```python
from build123d import *

# Parameters (mm, degrees)
SKETCH1_R               = 1.7526
BOSS_EXTRUDE1_DEPTH     = 20.240625
CUT_EXTRUDE1_START      = 17.4625
CUT_EXTRUDE1_DEPTH      = 6.35
CUT_EXTRUDE2_START      = -17.4625
CUT_EXTRUDE2_DEPTH      = 6.35
CUT_EXTRUDE3_DEPTH      = 40.737078408
CUT_EXTRUDE3_DEPTH_BACK = 40.737078408
SKETCH4_R               = 15.875


with BuildPart() as part:
    # Sketch1 → Boss-Extrude1 (new, symmetric)
    with BuildSketch(Plane.XY):
        with BuildLine():
            Line((0, 31.75), (12.7, 31.75))
            ThreePointArc((12.7, 31.75), (3.690995675, 0), (12.7, -31.75))
            Line((12.7, -31.75), (0, -31.75))
            ThreePointArc((0, -31.75), (-9.009004325, 0), (0, 31.75))
        make_face()
        with Locations((3.690995675, 25.4)):
            Circle(SKETCH1_R, mode=Mode.SUBTRACT)
        with Locations((3.690995675, -25.4)):
            Circle(SKETCH1_R, mode=Mode.SUBTRACT)
    extrude(amount=BOSS_EXTRUDE1_DEPTH, both=True)

    # Sketch2 → Cut-Extrude1 (cut)
    with BuildSketch(Plane.XY.offset(CUT_EXTRUDE1_START)):
        Polygon((21.851555668, 28.575), (1.85790857, 28.575), (0.024821465, 25.4), (1.85790857, 22.225), (21.851555668, 22.225), align=None)
        Polygon((21.851555668, -28.575), (21.851555668, -22.225), (1.85790857, -22.225), (0.024821465, -25.4), (1.85790857, -28.575), align=None)
    extrude(amount=-CUT_EXTRUDE1_DEPTH, mode=Mode.SUBTRACT)

    # Sketch2<2> → Cut-Extrude2 (cut)
    with BuildSketch(Plane.XY.offset(CUT_EXTRUDE2_START)):
        Polygon((21.851555668, 28.575), (1.85790857, 28.575), (0.024821465, 25.4), (1.85790857, 22.225), (21.851555668, 22.225), align=None)
        Polygon((21.851555668, -28.575), (21.851555668, -22.225), (1.85790857, -22.225), (0.024821465, -25.4), (1.85790857, -28.575), align=None)
    extrude(amount=CUT_EXTRUDE2_DEPTH, mode=Mode.SUBTRACT)

    # Sketch4 → Cut-Extrude3 (cut, two sides: drawn at the far end of the back side and taken through both)
    with BuildSketch(Plane(origin=(0, 0, 0), x_dir=(0, 0, -1), z_dir=(1, 0, 0)).offset(-CUT_EXTRUDE3_DEPTH_BACK)):
        Circle(SKETCH4_R)
    extrude(amount=CUT_EXTRUDE3_DEPTH + CUT_EXTRUDE3_DEPTH_BACK, mode=Mode.SUBTRACT)


solid = part.part
```
The model under review builds one solid part; all positions refer to its coordinate system, in mm. A direction names the side the tool comes from. Round coordinates to 2 decimals unless told otherwise and drop trailing zeros. Write each loop counter-clockwise with the first axis right and the second up, starting at its lowest first coordinate (ties: lowest second). Pieces come first, ordered by that corner, then holes. Notation, with made-up numbers: M 85,-33 L 134,-33 A21 cw 134,-16 Z; hole C 23.5,61.5 d7. An arc over 180 degrees is marked long. Use CSV: the item, a comma, the result in double quotes. Start each with the question number.
(1) We need section A-A, the plane y = 0. State the section outline as (x, z) points (3 decimals).
(2) For line 1 along Z through (x, y) = (6.75, -24.5); line 2 along Z through (x, y) = (-1, 0.5); line 3 along Y through (x, z) = (2.5, 5.5), list the stretches that pass through material, from the lowest coordinate up.
(3) We need section B-B, the plane z = 4.5. State the section outline as (x, y) points.
(4) Tool access review of faces 1 (the face through (5.623, 15.161, 9.279)), 2 (the face through (5, -27, 11.112)): name each direction out of +Z, -Z, +X, -X, +Y, -Y from which nothing blocks a thin tool from reaching the whole face with its end or side.
(5) We need section D-D, the plane z = 14. State the section outline as (x, y) points (3 decimals), then the cut area to 3 significant figures.
(6) The part is to be moulded in two halves that separate along X. For faces 3 (the face through (0.93, 23.83, 14.33)), 4 (the face through (3.31, -27.11, -0.16)), 5 (the face through (5, -22.225, 14)), say which applies: +X half, -X half, draft (parallel to the pull), parting line (faces both ways), or undercut.
(7) Clearance check with flat-ended pins moving along their axes: P1, Ø3, axis at x = -5.5, z = -13.5, coming from the -Y side; P2, Ø6, axis at y = 15, z = -12, coming from the +X side. State where each tip first meets the part, or that it passes through.
Findings:
1,outline,"M -9.009,-20.241 L 3.691,-20.241 L 3.691,-15.875 L -9.009,-15.875 Z; M -9.009,15.875 L 3.691,15.875 L 3.691,20.241 L -9.009,20.241 Z"
2,line 1,"-20.24 to -17.46, -11.11 to 11.11, 17.46 to 20.24"
2,line 2,"-20.24 to -15.87, 15.87 to 20.24"
2,line 3,"-31.75 to -26.69, -24.11 to -14.89, 14.89 to 24.11, 26.69 to 31.75"
3,outline,"M -7.06,-15.22 A60.45 ccw 0,-31.75 L 12.7,-31.75 A60.45 cw 5.64,-15.22 Z; M -7.06,15.22 L 5.64,15.22 A60.45 cw 12.7,31.75 L 0,31.75 A60.45 ccw Z; hole C 3.69,-25.4 d3.51; hole C 3.69,25.4 d3.51"
4,face 1,"+Z, -Z, +X"
4,face 2,"+X"
5,outline,"M -8.544,-7.484 A60.452 ccw 0,-31.75 L 12.7,-31.75 A60.452 cw 10.871,-28.575 L 1.858,-28.575 L 0.025,-25.4 L 1.858,-22.225 L 7.925,-22.225 A60.452 cw 4.156,-7.484 Z; M -8.544,7.484 L 4.156,7.484 A60.452 cw 7.925,22.225 L 1.858,22.225 L 0.025,25.4 L 1.858,28.575 L 10.871,28.575 A60.452 cw 12.7,31.75 L 0,31.75 A60.452 ccw Z"
5,area,"510 mm^2"
6,face 3,"+X half"
6,face 4,"undercut"
6,face 5,"draft"
7,P1,"y = -24.09"
7,P2,"x = 6.43"
